Build history of the part. All positions in model axes, mm. Face numbers are marked on the shaded views. A direction names the side the tool comes from. Round coordinates to 2 decimals unless told otherwise and drop trailing zeros. Loops run counter-clockwise (first coordinate to the right, second up) from the corner with the lowest first, then second, coordinate; pieces in that order, holes last.
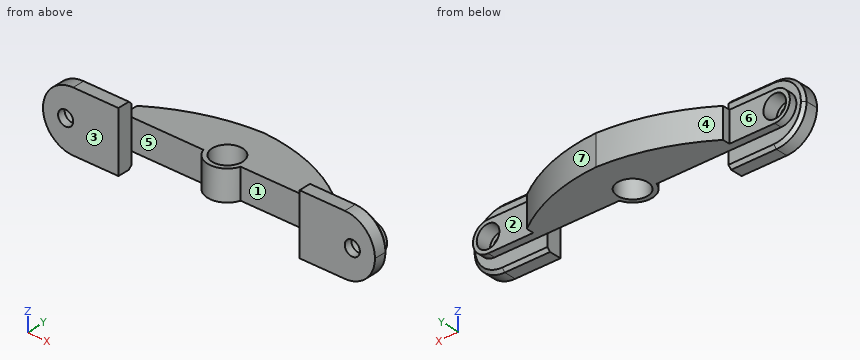
Autodesk Inventor part; units mm, degrees
ref_plane "Work Plane1" through (0, 0, -5) normal (0, 0, 1) x (1, 0, 0)
ref_plane "YZ Plane" through (0, 0, 0) normal (1, 0, 0) x (0, 1, 0)
ref_plane "XZ Plane" through (0, 0, 0) normal (0, 1, 0) x (-1, 0, 0)
sketch "Sketch1" plane through (0, 0, 0) normal (0, 1, 0) x (-1, 0, 0)
  line L0 (11, -8) -> (6, -8)
  line L1 (6, -8) -> (6, -4)
  line L2 (6, -4) -> (11, -4)
  line L3 (11, -4) -> (11, -8)
  line L4 (-6, -4) -> (-11, -4)
  line L5 (-11, -4) -> (-11, -8)
  line L6 (-11, -8) -> (-6, -8)
  line L7 (-6, -8) -> (-6, -4)
  point P0 (0, 0)
  dimension "d0" = 5
  dimension "d1" = 4
  dimension "d2" = 6
  dimension "d3" = 4
  dimension "d4" = 5
  dimension "d5" = 4
  dimension "d6" = 6
  dimension "d7" = 4
extrude "Extrusion1" add sketch "Sketch1" along normal blind 1
ref_plane "Work Plane1" through (0, 0, -5) normal (0, 0, 1) x (1, 0, 0)
sketch "Sketch3" plane through (0, 0, -5) normal (0, 0, 1) x (1, 0, 0)
  line L0 (11, 1) -> (11, 0)
  line L1 (11, 0) -> (6, 0)
  line L2 (6, 0) -> (6, 1)
  line L3 (6, 1) -> (11, 1)
  line L4 (-6, 1) -> (-6, 0)
  line L5 (-6, 0) -> (-11, 0)
  line L6 (-11, 0) -> (-11, 1)
  line L7 (-11, 1) -> (-6, 1)
  line L8 (-6, 1) -> (-11, 1)
  line L9 (6.5, 1) -> (6.5, 2)
  line L10 (-6.5, 2) -> (-6.5, 1)
  arc A0 (-1.2346, 1) -> (1.2346, 1) centre (0, 1.407) ccw
  line L11 (-6.5, 1) -> (-1.2346, 1)
  line L12 (1.2346, 1) -> (6.5, 1)
  arc A1 (0, 4.1975) -> (-6.5, 2) centre (0.6617, -8.4719) ccw
  arc A2 (6.5, 2) -> (0, 4.1975) centre (-0.3857, -7.6555) ccw
  line L13 (6.5, 2) -> (6, 2)
  line L14 (-6, 2) -> (-6.5, 2)
  point P0 (0, 0)
  point P1 (6, 1)
  dimension "d11" = 13
  dimension "d12" = 1
  dimension "d13" = 6.5
  dimension "d14" = 2.6
extrude "Extrusion2" add sketch "Sketch3" against normal blind 2 contours L3 L12 A0 L11 L7 L10 A1 A2 L9
sketch "Sketch4" plane through (0, 1, 0) normal (0, 1, 0) x (1, 0, 0)
  line L0 (0, 7) -> (-6.5, 7)
  line L1 (-6.5, 7) -> (-9.5, 7)
  line L2 (-9.5, 7) -> (-9.5, 5)
  line L3 (-9.5, 5) -> (-6.5, 5)
  line L4 (-6.5, 5) -> (-6.5, 7)
  arc A0 (-9.5, 7) -> (-9.5, 5) centre (-9.5, 6) ccw
  line L5 (6.5, 5) -> (6, 5)
  line L6 (6.5, 5) -> (9.5, 5)
  line L7 (9.5, 5) -> (9.5, 7)
  line L8 (9.5, 7) -> (6.5, 7)
  line L9 (6.5, 7) -> (6.5, 5)
  arc A1 (9.5, 5) -> (9.5, 7) centre (9.5, 6) ccw
  point P0 (0, 0)
  dimension "d17" = 3
  dimension "d18" = 2
  dimension "d19" = 1
  dimension "d20" = 3
  dimension "d21" = 2
  dimension "d22" = 1
extrude "Extrusion3" add sketch "Sketch4" along normal blind 0.5
sketch "Sketch5" plane through (0, 1.5, 0) normal (0, 1, 0) x (1, 0, 0)
  arc A0 (-9.5, 7) -> (-9.5, 5) centre (-9.5, 6) ccw
  point P0 (0, 0)
hole "Hole1" at (-9.5, 1.5, -6) direction (0, -1, 0) diameter 1 end through all counterbore diameter 1.5 counterbore depth 1
sketch "Sketch6" plane through (0, 1.5, 0) normal (0, 1, 0) x (1, 0, 0)
  arc A0 (9.5, 5) -> (9.5, 7) centre (9.5, 6) ccw
  point P0 (0, 0)
hole "Hole2" at (9.5, 1.5, -6) direction (0, -1, 0) diameter 1 end through all counterbore diameter 1.5 counterbore depth 1
sketch "Sketch7" plane through (0, 0, -5) normal (0, 0, 1) x (1, 0, 0)
  arc A0 (-1.2346, 1) -> (1.2346, 1) centre (0, 1.407) ccw
  point P0 (0, 0)
hole "Hole3" at (0, 1.407, -5) direction (0, 0, -1) diameter 2 end through all
fillet "Fillet1" radius 2 4 edges at (-11, 0.5, -4) (-11, 0.5, -8) (11, 0.5, -8) (11, 0.5, -4)
chamfer "Chamfer1" distance 0.2 angle 45 3 edges at (-7.5003, 1, -4) (-10.4144, 1, -4.5856) (-7.5003, 1, -8)
chamfer "Chamfer2" distance 0.2 angle 45 3 edges at (7.5002, 1, -4) (10.4144, 1, -7.4144) (7.5002, 1, -8)
properties part number "camfer,fillet dan holes"
(1) Slice it at A-A on x = 7.75. List the corners of the cut face in (y, z).
Responses:
outline: (0, -8) - (0.8, -8) - (1, -7.8) - (1, -7) - (1.5, -7) - (1.5, -5) - (1, -5) - (1, -4.2) - (0.8, -4) - (0, -4) - close
(2) Pull direction X, two halves, no side cores. Call the marked faces 4, 5, 6 and 7: +X half, -X half, draft (parallel to the pull), parting line (faces both ways), or undercut.
Responses:
face 4: -X half
face 5: undercut
face 6: draft
face 7: +X half
(3) Slice it at C-C on y = 3.3. List the corners of the cut face in (x, z).
Responses:
outline: (-4.07, -7) - (4.16, -7) - (4.16, -5) - (-4.07, -5) - close
(4) Which spindle directions (+Z, -Z, +X, -X, +Y, -Y) get a long thin tool onto all of the face, cutting with end or side? Do the marked faces 1, 2 and 3. Say none if no direction does.
Responses:
face 1: +Z, -Z, -Y
face 2: +Z, -Z, +X, +Y
face 3: +Z, -Z, +X, -X, -Y
(5) Pin check, flat tips, straight feed: P1, Ø1.2, axis at x = -9.5, z = -6, coming from the +Y side; P2, Ø1.2, axis at x = 3.5, y = 1.5, coming from the -Z side; P3, Ø1, axis at x = -1, z = -6, coming from the -Y side. Stop position of each tip, or through.
Responses:
P1: stops at y = 0.5
P2: stops at z = -7
P3: stops at y = 0.21
(6) Probe line 1 (Z direction, x = 9.5, y = 1.05); line 2 (X direction, y = 1.4, z = -5.8); line 3 (Y direction, x = 0, z = -6.05). List the from-to ranges inside material, lowest first.
Responses:
line 1: z = -7 to -6.75, -5.25 to -5
line 2: x = -10.48 to -10.22, -8.78 to -1, 1 to 8.78, 10.22 to 10.48
line 3: y = 0.11 to 0.41, 2.41 to 4.2
(7) Slice it at D-D on x = -5. List the corners of the cut face in (y, z), plus the area to 3 significant figures.
Responses:
outline: (1, -7) - (2.88, -7) - (2.88, -5) - (1, -5) - close
area: 3.76 mm2
(8) Slice it at B-B on x = 0.25. List the corners of the cut face in (y, z).
Responses:
outline: (0.13, -7) - (0.44, -7) - (0.44, -5) - (0.13, -5) - close; (2.38, -7) - (4.19, -7) - (4.19, -5) - (2.38, -5) - close
